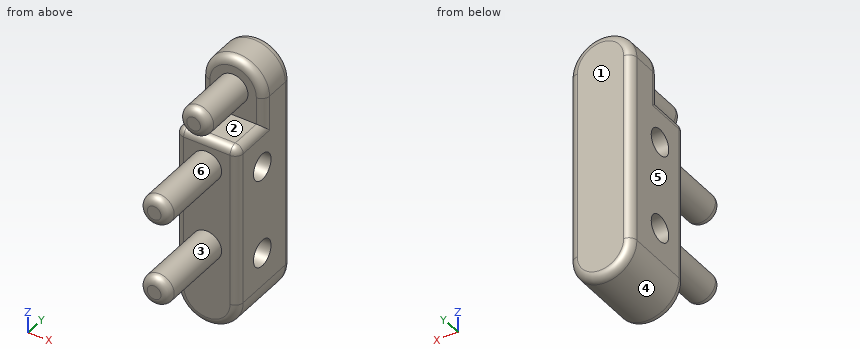
from build123d import *

# Parameters (mm, degrees)
F0_R     = 9.4597461698
F1_DEPTH = 101.6
F0_W     = 39.8592872384
F0_H     = 103.9333879682
F2_DEPTH = 50.8
F3_DEPTH = 25.4
F4_DEPTH = 63.5
F5_R     = 5.08
F6_R     = 5.08
F7_R     = 5.08
F8_R     = 8.4595796919
F9_DEPTH = 25.4
F12_R    = 5.08


# Not quite as in the source:
# - the program builds the solid bodies; features that only make, move or delete a surface that nothing else refers to are left out


with BuildPart() as f1:
    # F0 (on Front) → F1 (new body)
    with BuildSketch(Plane.XZ):
        with Locations((0, -35.6362370717)):
            Circle(F0_R)
    extrude(amount=F1_DEPTH)



with BuildPart() as f1b:
    # F0 (on Front) → F1, piece 2 (new body)
    with BuildSketch(Plane.XZ):
        with Locations((0, -88.4090361273)):
            Circle(F0_R)
    extrude(amount=F1_DEPTH)


with BuildPart() as f1_1:
    add(f1.part)

    add(f1b.part)  # F2 merges F1b
    # F0 (on Front) → F2 (join)
    with BuildSketch(Plane.XZ):
        with Locations((0, -69.4868988952)):
            Rectangle(F0_W, F0_H)
        with Locations((0, -88.4090361273)):
            Circle(F0_R, mode=Mode.SUBTRACT)
        with Locations((0, -35.6362370717)):
            Circle(F0_R, mode=Mode.SUBTRACT)
        with BuildLine():
            ThreePointArc((-19.9296436192, -121.4535928793), (0, -141.3832364985), (19.9296436192, -121.4535928793))
            Line((19.9296436192, -121.4535928793), (-19.9296436192, -121.4535928793))
        make_face()
    extrude(amount=F2_DEPTH)

    # F0 (on Front) → F3 (join)
    with BuildSketch(Plane.XZ):
        with BuildLine():
            Line((19.9296436192, -17.5202049111), (19.9296436192, 0))
            ThreePointArc((19.9296436192, 0), (0, 19.9296436192), (-19.9296436192, 0))
            Line((-19.9296436192, 0), (-19.9296436192, -17.5202049111))
            Line((-19.9296436192, -17.5202049111), (19.9296436192, -17.5202049111))
        make_face()
        Circle(F0_R, mode=Mode.SUBTRACT)
    extrude(amount=F3_DEPTH)

    # F0 (on Front) → F4 (join)
    with BuildSketch(Plane.XZ):
        Circle(F0_R)
    extrude(amount=F4_DEPTH)

    # F5
    f5_edges = [f1_1.edges().sort_by_distance(p)[0] for p in [
        (-19.929644, -50.8, -69.486899),
        (-19.929644, -38.1, -17.520205),
        (19.929644, -50.8, -69.486899),
        (0, -50.8, -17.520205),
        (19.929644, -38.1, -17.520205),
    ]]
    fillet(f5_edges, radius=F5_R)

    # F6
    f6_edges = [f1_1.edges().sort_by_distance(p)[0] for p in [
        (19.929644, 0, -60.726796),
        (0, 0, 19.929644),
        (-19.929644, 0, -60.726796),
        (0, 0, -141.383236),
    ]]
    fillet(f6_edges, radius=F6_R)

    # F7
    f7_edges = [f1_1.edges().sort_by_distance(p)[0] for p in [
        (-19.929644, -25.4, -8.760102),
        (-19.929644, -25.4, -20.060205),
        (0, -25.4, 19.929644),
        (19.929644, -15.24, 0),
    ]]
    fillet(f7_edges, radius=F7_R)

    # F8 (on Right) → F9 (cut, symmetric)
    with BuildSketch(Plane.YZ):
        with Locations((-27.3456163704, -42.5785966218)):
            Circle(F8_R)
        with Locations((-27.3456163704, -99.8373031616)):
            Circle(F8_R)
    extrude(amount=F9_DEPTH, both=True, mode=Mode.SUBTRACT)

    # F12
    f12_edges = [f1_1.edges().sort_by_distance(p)[0] for p in [
        (-9.459746, -101.6, -88.409036),
        (-9.459746, -101.6, -35.636237),
        (-9.459746, -63.5, 0),
    ]]
    fillet(f12_edges, radius=F12_R)


solid = f1_1.part
Input: part model. Units: mm. Frame: model coordinates. Face numbers are marked on the shaded views. A direction names the side the tool comes from. Coordinates: 2 decimals unless noted, no trailing zeros. Order: outer loops, then holes, each group sorted by start corner. A loop starts at its lowest first (then second) coordinate and runs counter-clockwise, first axis right, second up. Notation, with made-up numbers: M 73,0 L 88,0 A24 ccw 88,29 Z; hole C 83.5,14.5 d3. An arc over 180 degrees is marked long. Write item = value, one per line. Start each with the question number.
(1) Section A-A on y = -32.5. Output: boundary loops of the cut face in (x, z).
(2) Line query: line 1 along Z through (x, y) = (6, -23); line 2 along Z through (x, y) = (3, -35); line 3 along Z through (x, y) = (16, -30.5). Output: solid intervals per line, ascending. Write a range as [from, to].
(3) Section C-C on y = -9.5. Output: boundary loops of the cut face in (x, z), and give its area (3 significant figures).
(4) Pull-direction query (Z, two-part tool) for the marked faces 4, 5 and 6; classes: released by +Z, released by -Z, zero draft, split by the parting line, or undercut.
(5) Reachability of the marked faces 1, 2 and 3 from +Z, -Z, +X, -X, +Y, -Y: full face, straight path, thin tool, end or side. Return the list, or none.
(6) Section D-D on x = 0. Give the number of separate pieces and of enclosed holes in the cut face, and give its area (3 significant figures).
(7) Section B-B on z = -67. Output: boundary loops of the cut face in (x, y), and give its area (3 significant figures).
(8) First-contact query: P1, Ø9, axis at x = 6.5, z = -69.5, coming from the -Y side; P2, Ø4.5, axis at x = 1.5, z = -0.5, coming from the -Y side; P3, Ø5, axis at x = -11, y = -15.5, coming from the +Z side. Flat tips, straight axial feed; report the tip coordinate or a pass-through.
Result set:
q1.outline = M -19.93,-121.45 A19.93 ccw 19.93,-121.45 L 19.93,-106.55 L -19.93,-106.55 Z; M -19.93,-93.13 L 19.93,-93.13 L 19.93,-49.29 L -19.93,-49.29 Z; M -19.93,-35.87 L 19.93,-35.87 L 19.93,-22.6 A5.08 ccw 14.85,-17.52 L -14.85,-17.52 A5.08 ccw -19.93,-22.6 Z; C 0,0 d18.92
q2.line_1 = [-140.46, -107.1], [-92.58, -49.84], [-35.32, 18.2]
q2.line_2 = [-141.16, -103.44], [-96.24, -46.18], [-38.98, -17.52], [-8.97, 8.97]
q2.line_3 = [-133.34, -107.69], [-91.99, -50.43], [-34.73, -17.65]
q3.outline = M -19.93,-121.45 A19.93 ccw 19.93,-121.45 L 19.93,0 A19.93 ccw -19.93,0 Z
q3.area = 6,090 mm²
q4.face_4 = released by -Z
q4.face_5 = zero draft
q4.face_6 = undercut
q5.face_1 = +Z, -Z, +X, -X, +Y
q5.face_2 = +X, -X, -Y
q5.face_3 = -Y
q6.separate_pieces = 1
q6.enclosed_holes = 2
q6.area = 9,380 mm²
q7.outline = M -19.93,-45.72 A5.08 ccw -14.85,-50.8 L 14.85,-50.8 A5.08 ccw 19.93,-45.72 L 19.93,-5.08 A5.08 ccw 14.85,0 L -14.85,0 A5.08 ccw -19.93,-5.08 Z
q7.area = 2,000 mm²
q8.P1 = -50.8
q8.P2 = -63.5
q8.P3 = 18.03
